```python
from build123d import *

# Parameters (mm, degrees)
F1_DEPTH = 11
F0_R     = 2
F2_DEPTH = 3
F3_R     = 5
F4_R     = 1


with BuildPart() as f1:
    # F0 (on Top) → F1 (new body)
    with BuildSketch(Plane.XY):
        with BuildLine():
            Line((-40, 0), (0, 0))
            Line((0, 0), (0, 40))
            Line((0, 40), (-2.5865715742, 40))
            Line((-2.5865715742, 40), (-2.5865715742, 20.0865715742))
            ThreePointArc((-2.5865715742, 20.0865715742), (-20.0865715742, 2.5865715742), (-37.5865715742, 20.0865715742))
            Line((-37.5865715742, 20.0865715742), (-37.5865715742, 40))
            Line((-37.5865715742, 40), (-40, 40))
            Line((-40, 40), (-40, 0))
        make_face()
    extrude(amount=F1_DEPTH)

    # F0 (on Top) → F2 (join)
    with BuildSketch(Plane.XY):
        with BuildLine():
            Line((-2.5865715742, 20.0865715742), (-2.5865715742, 40))
            Line((-2.5865715742, 40), (-37.5865715742, 40))
            Line((-37.5865715742, 40), (-37.5865715742, 20.0865715742))
            ThreePointArc((-37.5865715742, 20.0865715742), (-20.0865715742, 37.5865715742), (-2.5865715742, 20.0865715742))
        make_face()
        with BuildLine():
            ThreePointArc((-37.5865715742, 20.0865715742), (-20.0865715742, 2.5865715742), (-2.5865715742, 20.0865715742))
            ThreePointArc((-2.5865715742, 20.0865715742), (-20.0865715742, 37.5865715742), (-37.5865715742, 20.0865715742))
        make_face()
        with Locations((-20.0865715742, 20.0865715742)):
            Circle(F0_R, mode=Mode.SUBTRACT)
    extrude(amount=F2_DEPTH)

    # F3
    f3_edges = [f1.edges().sort_by_distance(p)[0] for p in [
        (-40, 0, 5.5),
        (0, 0, 5.5),
        (0, 40, 5.5),
        (-40, 40, 5.5),
    ]]
    fillet(f3_edges, radius=F3_R)

    # F4
    f4_edges = [f1.edges().sort_by_distance(p)[0] for p in [
        (-20.086572, 2.586572, 11),
        (-37.586572, 29.682774, 11),
        (-2.586572, 39.378968, 7),
        (-37.586572, 39.278977, 7),
    ]]
    fillet(f4_edges, radius=F4_R)


solid = f1.part
```
Design review of the part built by this model. Coordinates are the model's own, in mm. A direction names the side the tool comes from. Give positions to 0.01 mm unless a question says otherwise; leave off trailing zeros. Write each loop counter-clockwise with the first axis right and the second up, starting at its lowest first coordinate (ties: lowest second). Pieces come first, ordered by that corner, then holes. Notation, with made-up numbers: (83.5, 27.5) - (116.5, 27.5) arc R15 ccw to (116.5, 32.5) - close; hole circle Ø8 at (-13, 14). An arc over 180 degrees is marked (long way). Return JSON: item names as keys, results as strings. Group by question number.
(1) We need section A-A, the plane z = 2. Give the boundary of the cut face in (x, y).
(2) We need section C-C, the plane z = 6.5. Give the boundary of the cut face in (x, y), then the cut area to 3 significant figures.
(3) Insertion check: pin 1 (6 mm diameter, centred on x = -32, z = 9, fed in from +Y); pin 2 (1.5 mm diameter, centred on y = 35.5, z = 8, fed in from -X); pin 3 (6 mm diameter, centred on x = -24, y = 31, fed in from +Z). Each pin has a flat end and moves straight along its axis. Give the tip position at first contact, or say it passes through.
(4) To check wall thickness, follow probe 1 along X at (y, z) = (31, 9.5); probe 2 along Z at (x, y) = (-23.5, 8); probe 3 along X at (y, z) = (6, 4). State the ranges of each line that lie inside material, in increasing order.
(5) We need section B-B, the plane y = 34.5. Give the boundary of the cut face in (x, z), then the cut area to 3 significant figures.
(6) Mouldability with a two-part tool opening along X and no side actions: class faces 3 (the cylindrical face through (-19.7, 2.59, 6.45)), 4 (the cylindrical face through (-39, 2, 6)), 5 (the flat face through (-20, 0, 5)) as +X half, -X half, draft (parallel to the pull), parting line (faces both ways), or undercut.
(7) Machinability: for faces 1 (the cylindrical face through (-37.887, 29.053, 10.715)), 2 (the flat face through (-40, 20, 5)), which of the approach directions +Z, -Z, +X, -X, +Y, -Y give a long, thin tool a straight path to every point of the face, cutting with its end or side? Answer none if there is none.
Reported:
{
 "1": {"outline": "(-40, 5) arc R5 ccw to (-35, 0) - (-5, 0) arc R5 ccw to (0, 5) - (0, 35) arc R5 ccw to (-5, 40) - (-35, 40) arc R5 ccw to (-40, 35) - close; hole circle Ø4 at (-20.09, 20.09)"},
 "2": {"outline": "(-40, 5) arc R5 ccw to (-35, 0) - (-5, 0) arc R5 ccw to (0, 5) - (0, 35) arc R5 ccw to (-0.73, 37.61) arc R1 ccw to (-2.59, 37.09) - (-2.59, 20.09) arc R17.5 cw to (-37.59, 20.09) - (-37.59, 36.77) arc R1 ccw to (-39.48, 37.21) arc R5 ccw to (-40, 35) - close", "area": "399 mm2"},
 "3": {"pin 1": "stops at y = 10.93", "pin 2": "stops at x = -40", "pin 3": "stops at z = 3"},
 "4": {"probe 1": "x = -40 to -37.59, -2.59 to 0", "probe 2": "z = 0 to 3", "probe 3": "x = -40 to -30.47, -9.7 to 0"},
 "5": {"outline": "(-40, 0) - (0, 0) - (0, 11) - (-1.59, 11) arc R1 ccw to (-2.59, 10) - (-2.59, 3) - (-37.59, 3) - (-37.59, 10) arc R1 ccw to (-38.59, 11) - (-40, 11) - close", "area": "160 mm2"},
 "6": {"face 3": "undercut", "face 4": "-X half", "face 5": "draft"},
 "7": {"face 1": "+Z, +Y", "face 2": "+Z, -Z, -X, +Y, -Y"}
}
